Source: three-view drawing plus pictorial views. Frame: mm from the lowest corner of the part. A direction names the side the tool comes from. Give positions to 0.01 mm unless a question says otherwise; leave off trailing zeros. Order: outer loops, then holes, each group sorted by start corner. A loop starts at its lowest first (then second) coordinate and runs counter-clockwise, first axis right, second up. Notation, with made-up numbers: M 0.5,56 L 22.5,56 A9 ccw 22.5,63 Z; hole C -14.5,56 d11. An arc over 180 degrees is marked long. One line per question, with ' | ' between items. Start each with the question number.
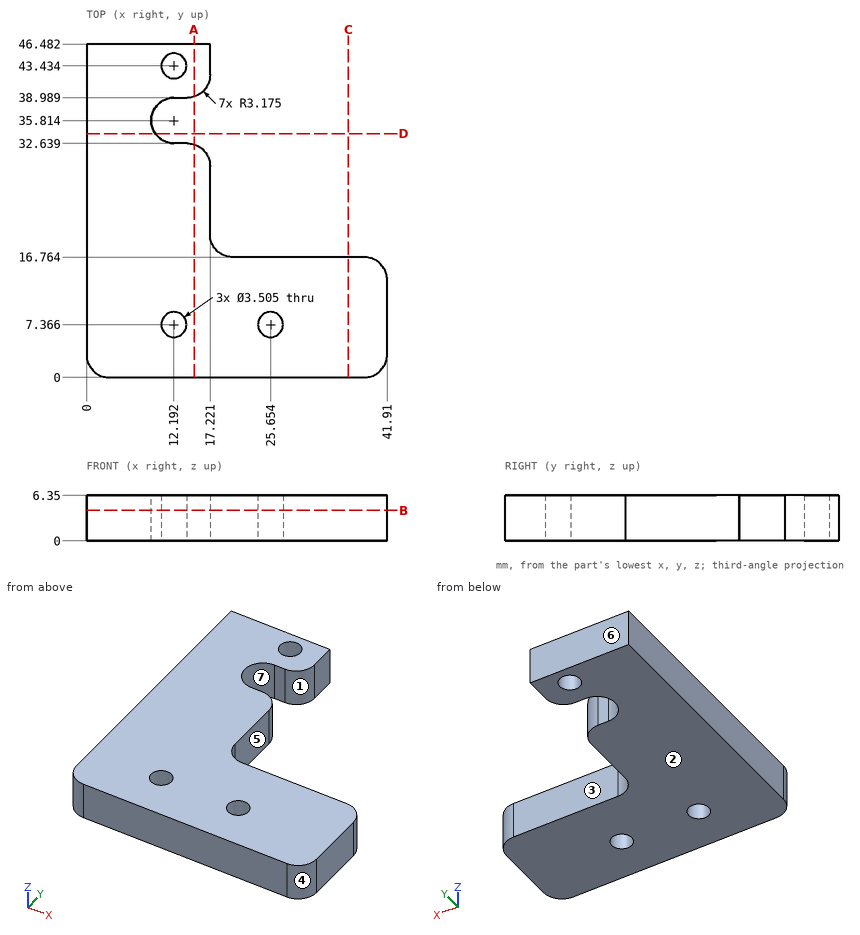
Item 1: Pin query (flat end, axial travel): pin 1 Ø3 at (x, z) = (32.5, 3) entering from +Y; pin 2 Ø2 at (y, z) = (43.5, 4) entering from +X. Return the tip coordinate at first contact, or that it passes through.
Item 2: Cut plane D-D on y = 34. Return the cut outline in (x, z), and give its area (3 significant figures).
Item 3: Cut plane B-B on z = 4.25. Count the separate pieces of the cut face and the enclosed holes in it, and give its area (3 significant figures).
Item 4: Reachability of the marked faces 1, 2 and 3 from +Z, -Z, +X, -X, +Y, -Y: full face, straight path, thin tool, end or side. Return the list, or none.
Item 5: Mould query, pull axis Y, two halves, no side actions, for the marked faces 4, 5, 6 and 7. Classes: pulls with the +Y half, pulls with the -Y half, needs draft (parallel to the pull), parting line crosses it, or undercut.
Item 6: Cut plane A-A on x = 15. Return the cut outline in (y, z), and give its area (3 significant figures).
Item 7: Line query: line 1 (X direction, y = 36, z = 1.75); line 2 (X direction, y = 29.5, z = 3); line 3 (X direction, y = 7, z = 0.5). Output: solid intervals per line, ascending.
Item 8: Cut plane C-C on x = 36.5. Return the cut outline in (y, z), and give its area (3 significant figures).
Results are:
1) pin 1: stops at y = 16.76 | pin 2: stops at x = 17.22
2) outline: M 0,0 L 9.59,0 L 9.59,6.35 L 0,6.35 Z | area: 60.9 mm2
3) separate pieces: 1 | enclosed holes: 3 | area: 1,130 mm2
4) face 1: +Z, -Z, +X | face 2: -Z, +X, -X, +Y, -Y | face 3: +Z, -Z, +X, +Y
5) face 4: pulls with the -Y half | face 5: needs draft | face 6: pulls with the +Y half | face 7: undercut
6) outline: M 0,0 L 32.49,0 L 32.49,6.35 L 0,6.35 Z; M 39.14,0 L 46.48,0 L 46.48,6.35 L 39.14,6.35 Z | area: 253 mm2
7) line 1: x = 0 to 9.02 | line 2: x = 0 to 17.22 | line 3: x = 0 to 10.48, 13.91 to 23.94, 27.37 to 41.91
8) outline: M 0,0 L 16.76,0 L 16.76,6.35 L 0,6.35 Z | area: 106 mm2
